Geometry: see drawing. Coordinates: mm, zero at the bounding-box minimum. Give positions to 0.01 mm unless a question says otherwise; leave off trailing zeros. Write each loop counter-clockwise with the first axis right and the second up, starting at its lowest first coordinate (ties: lowest second). Pieces come first, ordered by that corner, then holes. Notation, with made-up numbers: M 84,63.5 L 125,63.5 A24 ccw 125,87.5 Z; hole C 83.25,57 d7. An arc over 180 degrees is marked long. Answer as a JSON object with one key per item and string values. Group by question number.
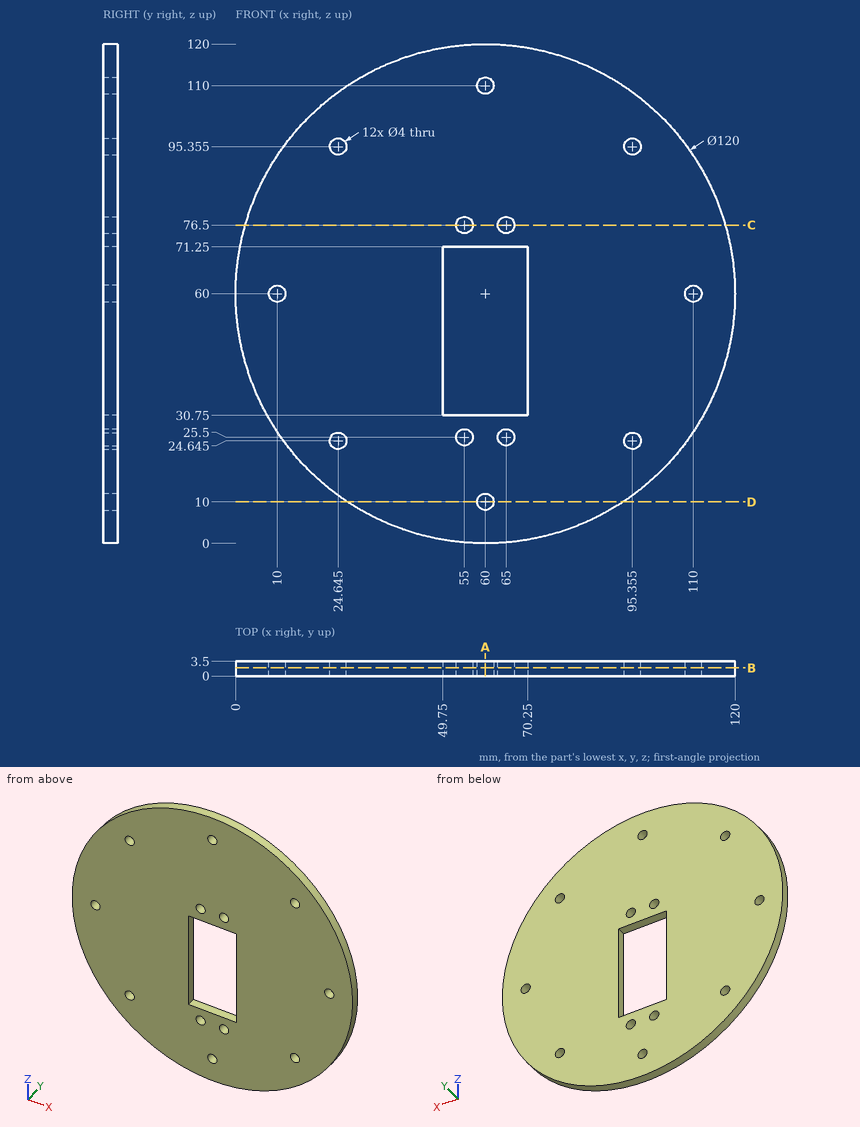
(1) Section C-C, the plane z = 76.5. Return loops of the section in (x, y), plus the area to 3 significant figures.
(2) Section D-D, the plane z = 10. Return loops of the section in (x, y), plus the area to 3 significant figures.
(3) Section A-A, the plane x = 60. Return loops of the section in (y, z), plus the area to 3 significant figures.
(4) Contact query for flat-ended pins moving along their axis: pin 1 Ø2 at (y, z) = (1, 65.5) entering from +X; pin 2 Ø1.5 at (y, z) = (2.5, 27.5) entering from +X; pin 3 Ø1.5 at (y, z) = (3, 93) entering from +X (1 decimal). Output: stop coordinate, or through.
(5) Ray query, L1, parallel to Z at x = 55, y = 1.75; L2, parallel to X at y = 2.7, z = 111 (1 decimal); L3, parallel to Z at x = 95, y = 1.75 (1 decimal). Return the intervals inside material, ascending. Write a range as [from, to].
(6) Section B-B, the plane y = 1.95. State how many separate pieces and enclosed holes the cut face has, plus the area to 3 significant figures.
Reported:
{
 "1": {"outline": "M 2.31,0 L 53,0 L 53,3.5 L 2.31,3.5 Z; M 57,0 L 63,0 L 63,3.5 L 57,3.5 Z; M 67,0 L 117.69,0 L 117.69,3.5 L 67,3.5 Z", "area": "376 mm2"},
 "2": {"outline": "M 26.83,0 L 58,0 L 58,3.5 L 26.83,3.5 Z; M 62,0 L 93.17,0 L 93.17,3.5 L 62,3.5 Z", "area": "218 mm2"},
 "3": {"outline": "M 0,0 L 3.5,0 L 3.5,8 L 0,8 Z; M 0,12 L 3.5,12 L 3.5,30.75 L 0,30.75 Z; M 0,71.25 L 3.5,71.25 L 3.5,108 L 0,108 Z; M 0,112 L 3.5,112 L 3.5,120 L 0,120 Z", "area": "250 mm2"},
 "4": {"pin 1": "stops at x = 119.83", "pin 2": "stops at x = 110.91", "pin 3": "stops at x = 110.6"},
 "5": {"L1": "z = [0.21, 23.5], [27.5, 30.75], [71.25, 74.5], [78.5, 119.79]", "L2": "x = [28.4, 58.3], [61.7, 91.6]", "L3": "z = [11.3, 22.7], [26.6, 93.4], [97.3, 108.7]"},
 "6": {"separate pieces": "1", "enclosed holes": "13", "area": "10,300 mm2"}
}
